Geometry: see drawing. Coordinates: mm, zero at the bounding-box minimum. Give positions to 0.01 mm unless a question says otherwise; leave off trailing zeros. Write each loop counter-clockwise with the first axis right and the second up, starting at its lowest first coordinate (ties: lowest second). Pieces come first, ordered by that corner, then holes. Notation, with made-up numbers: (45, 48.5) - (69, 48.5) arc R33 ccw to (69, 80.5) - close; hole circle Ø5 at (16, 11). An arc over 180 degrees is marked (long way). One line per question, with ' | ' between items. Start each with the question number.
(1) Section C-C, the plane x = 15. Return loops of the section in (y, z).
(2) Section B-B, the plane y = 0.4. Return loops of the section in (x, z).
(3) Section A-A, the plane z = 19.75. Return loops of the section in (x, y).
(4) Ray query, line 1 (X direction, y = 0.7, z = 21.25); line 2 (Z direction, x = 15, y = 0.3); line 3 (Z direction, x = 2.25, y = 0.1). Return the intervals inside material, ascending. Write a range as [from, to].
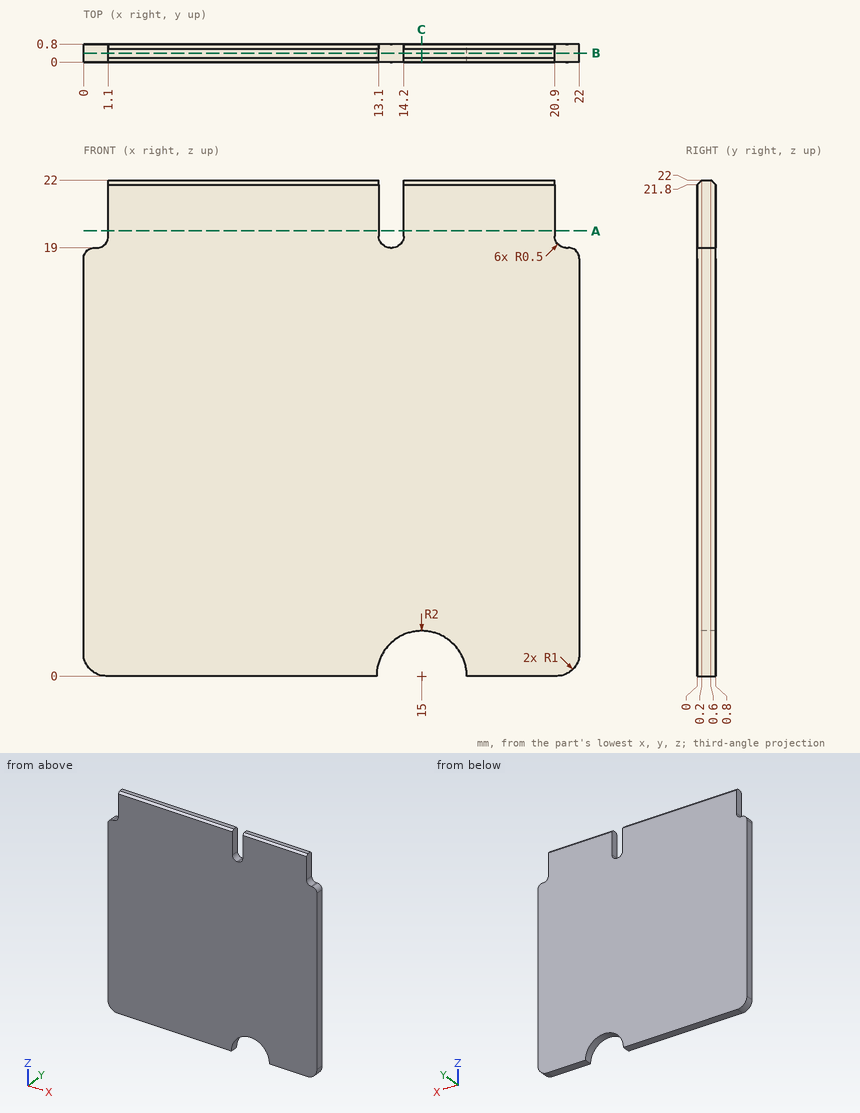
Check sheet entries:
1) outline: (0, 2) - (0.8, 2) - (0.8, 21.8) - (0.6, 22) - (0.2, 22) - (0, 21.8) - close
2) outline: (0, 1) arc R1 ccw to (1, 0) - (13, 0) arc R2 cw to (17, 0) - (21, 0) arc R1 ccw to (22, 1) - (22, 18.5) arc R0.5 ccw to (21.5, 19) - (21.4, 19) arc R0.5 cw to (20.9, 19.5) - (20.9, 22) - (14.2, 22) - (14.2, 19.5) arc R0.5 cw to (13.7, 19) - (13.6, 19) arc R0.5 cw to (13.1, 19.5) - (13.1, 22) - (1.1, 22) - (1.1, 19.5) arc R0.5 cw to (0.6, 19) - (0.5, 19) arc R0.5 ccw to (0, 18.5) - close
3) outline: (1.1, 0) - (13.1, 0) - (13.1, 0.8) - (1.1, 0.8) - close; (14.2, 0) - (20.9, 0) - (20.9, 0.8) - (14.2, 0.8) - close
4) line 1: [1.1, 13.1], [14.2, 20.9] | line 2: [2, 22] | line 3: [0, 21.9]
